from build123d import *

# Parameters (mm, degrees)
SKETCH1_W           = 100
SKETCH1_H           = 36
BOSS_EXTRUDE1_DEPTH = 4
SKETCH5_W           = 80
SKETCH5_H           = 15
BOSS_EXTRUDE3_DEPTH = 4
SKETCH6_R           = 1.25
CUT_EXTRUDE3_DEPTH  = 56.722526863
FILLET3_R           = 2.5
FILLET4_R           = 2.5
FILLET5_R           = 10
SKETCH7_R           = 1.6
CUT_EXTRUDE4_DEPTH  = 4


with BuildPart() as part:
    # Sketch1 → Boss-Extrude1 (new body)
    with BuildSketch(Plane.XY):
        Rectangle(SKETCH1_W, SKETCH1_H)
    extrude(amount=BOSS_EXTRUDE1_DEPTH)

    # Sketch5 → Boss-Extrude3 (add)
    with BuildSketch(Plane.XZ.offset(18)):
        with Locations((0, 7.5)):
            Rectangle(SKETCH5_W, SKETCH5_H)
    extrude(amount=BOSS_EXTRUDE3_DEPTH)

    # Sketch6 → Cut-Extrude3 (cut, through all)
    with BuildSketch(Plane.XY.offset(4)):
        with Locations((35, 3)):
            Circle(SKETCH6_R)
        with Locations((-35, 3)):
            Circle(SKETCH6_R)
    extrude(amount=-CUT_EXTRUDE3_DEPTH, mode=Mode.SUBTRACT)

    # Fillet3
    fillet3_edges = [part.edges().sort_by_distance(p)[0] for p in [
        (0, -18, 4),
    ]]
    fillet(fillet3_edges, radius=FILLET3_R)

    # Fillet4
    fillet4_edges = [part.edges().sort_by_distance(p)[0] for p in [
        (-40, -18, 2),
        (40, -18, 2),
    ]]
    fillet(fillet4_edges, radius=FILLET4_R)

    # Fillet5
    fillet5_edges = [part.edges().sort_by_distance(p)[0] for p in [
        (-50, -18, 2),
        (50, -18, 2),
        (-50, 18, 2),
        (50, 18, 2),
    ]]
    fillet(fillet5_edges, radius=FILLET5_R)

    # Sketch7 → Cut-Extrude4 (cut)
    with BuildSketch(Plane.XZ.offset(22)):
        with Locations(Location((33, 11, 0), (0, 0, 270))):
            Circle(SKETCH7_R)
        with Locations(Location((-33, 11, 0), (0, 0, 270))):
            Circle(SKETCH7_R)
    extrude(amount=-CUT_EXTRUDE4_DEPTH, mode=Mode.SUBTRACT)


solid = part.part
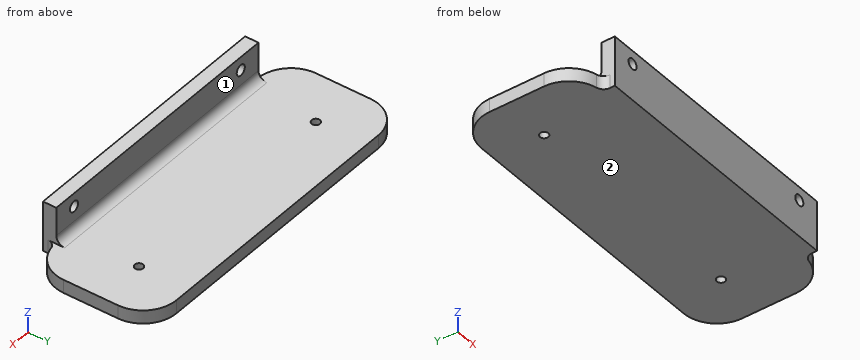
Could you check a few things on this model? Use its own coordinates, in mm. Face numbers are marked on the shaded views. A direction names the side the tool comes from. Give positions to 0.01 mm unless a question says otherwise; leave off trailing zeros. Loops run counter-clockwise (first coordinate to the right, second up) from the corner with the lowest first, then second, coordinate; pieces in that order, holes last. Notation, with made-up numbers: (46, 7) -> (90, 7) arc R19 cw to (90, 26) -> close; hole circle Ø10 at (14.25, -27.5). An arc over 180 degrees is marked (long way). Return JSON: item names as keys, results as strings.
Item 1: I'm going to push flat-ended pins straight in: pin 1 (2 mm diameter, centred on y = -19.5, z = 10, fed in from -X); pin 2 (3.5 mm diameter, centred on x = 33, z = 11, fed in from +Y); pin 3 (11.5 mm diameter, centred on x = 3.5, y = -7.5, fed in from +Z). Where does each tip first touch, or does it pass through?
Geometry results:
{"pin 1": "stops at x = -40", "pin 2": "stops at y = -18", "pin 3": "stops at z = 4"}
Item 2: If we section it at B-B on y = 3: List the corners of the cut face in (x, z) for me.
Geometry results:
{"outline": "(-50, 0) -> (-36.25, 0) -> (-36.25, 4) -> (-50, 4) -> close; (-33.75, 0) -> (33.75, 0) -> (33.75, 4) -> (-33.75, 4) -> close; (36.25, 0) -> (50, 0) -> (50, 4) -> (36.25, 4) -> close"}
Item 3: I need wall thicknesses on L1, parallel to X at y = -20.25, z = 11; L2, parallel to Y at x = -35, z = 2.75; L3, parallel to Z at x = 28, y = -11.5. Which ranges of each line are inside material? Lowest first, please. Write a range as from..to.
Geometry results:
{"L1": "x = -40..-34.6, -31.4..31.4, 34.6..40", "L2": "y = -22..1.75, 4.25..18", "L3": "z = 0..4"}
Item 4: Which directions (+Z, -Z, +X, -X, +Y, -Y) give clear straight access to the entire face, cutting with the end or side of a thin tool? Please do the marked faces 1 and 2.
Geometry results:
{"face 1": "+Z, +X, -X, +Y", "face 2": "-Z, +X, -X, +Y, -Y"}
Item 5: If we section it at A-A on z = 11: List the corners of the cut face in (x, y) for me.
Geometry results:
{"outline": "(-40, -22) -> (-34.6, -22) -> (-34.6, -18) -> (-40, -18) -> close; (-31.4, -22) -> (31.4, -22) -> (31.4, -18) -> (-31.4, -18) -> close; (34.6, -22) -> (40, -22) -> (40, -18) -> (34.6, -18) -> close"}
Item 6: If we section it at C-C on x = -14: List the corners of the cut face in (y, z) for me, plus the area to 3 significant figures.
Geometry results:
{"outline": "(-22, 0) -> (18, 0) -> (18, 4) -> (-15.5, 4) arc R2.5 cw to (-18, 6.5) -> (-18, 15) -> (-22, 15) -> close", "area": "205 mm²"}
Item 7: If we section it at D-D on z = 1.5: Count the separate pieces of the cut face and the enclosed holes in it, plus the area to 3 significant figures.
Geometry results:
{"separate pieces": "1", "enclosed holes": "2", "area": "3,830 mm²"}
